For this review, take the finished solid that the model builds, in its own axes (mm). Give positions to 0.01 mm unless a question says otherwise; leave off trailing zeros. Order: outer loops, then holes, each group sorted by start corner. A loop starts at its lowest first (then second) coordinate and runs counter-clockwise, first axis right, second up.
Item 1: Consider section C-C (y = 136). Give the boundary of the cut face in (x, z).
Item 2: Consider section A-A (x = -201.93). Give the boundary of the cut face in (y, z).
Item 3: Consider section B-B (y = 90.5). Give the boundary of the cut face in (x, z), plus the area to 3 significant figures.
Item 4: Consider section D-D (x = -115). Give the boundary of the cut face in (y, z).
Item 5: For probe 1 along Y at (x, z) = (-151.13, 1.85); probe 2 along Y at (x, z) = (-74.93, 1.95); probe 3 along X at (y, z) = (216, 0.95), list the stretches that pass through material, from the lowest coordinate up.
```python
from build123d import *

# Parameters (mm, degrees)
SKETCH1_W               = 228.6
SKETCH1_H               = 228.6
BOSS_EXTRUDE1_DEPTH     = 2.54
SKETCH4_R               = 19.05
CUT_EXTRUDE2_DEPTH      = 378.179309613
FILL_PATTERN2_OUTLINE_R = 19.05
FILL_PATTERN2_DEPTH     = 2.54


# Read off the part's stored shape, not the designer's step: Fill Pattern2
with BuildPart() as part:
    # Sketch1 → Boss-Extrude1 (new body)
    with BuildSketch(Plane.XY):
        with Locations((-152.4, 152.4)):
            Rectangle(SKETCH1_W, SKETCH1_H)
    extrude(amount=BOSS_EXTRUDE1_DEPTH)

    # Sketch4 → Cut-Extrude2 (cut, through all)
    with BuildSketch(Plane.XY):
        with Locations((-227.33, 218.44)):
            Circle(SKETCH4_R)
    extrude(amount=CUT_EXTRUDE2_DEPTH, mode=Mode.SUBTRACT)

    # Fill Pattern2 outline → Fill Pattern2 (cut)
    with BuildSketch(Plane.XY):
        with Locations((-74.93, 130.451818976)):
            Circle(FILL_PATTERN2_OUTLINE_R)
        with Locations((-201.93, 86.457728463)):
            Circle(FILL_PATTERN2_OUTLINE_R)
        with Locations((-176.53, 218.44)):
            Circle(FILL_PATTERN2_OUTLINE_R)
        with Locations((-201.93, 174.445909488)):
            Circle(FILL_PATTERN2_OUTLINE_R)
        with Locations((-227.33, 130.451818976)):
            Circle(FILL_PATTERN2_OUTLINE_R)
        with Locations((-125.73, 130.451818976)):
            Circle(FILL_PATTERN2_OUTLINE_R)
        with Locations((-100.33, 174.445909488)):
            Circle(FILL_PATTERN2_OUTLINE_R)
        with Locations((-74.93, 218.44)):
            Circle(FILL_PATTERN2_OUTLINE_R)
        with Locations((-100.33, 86.457728463)):
            Circle(FILL_PATTERN2_OUTLINE_R)
        with Locations((-176.53, 130.451818976)):
            Circle(FILL_PATTERN2_OUTLINE_R)
        with Locations((-151.13, 174.445909488)):
            Circle(FILL_PATTERN2_OUTLINE_R)
        with Locations((-125.73, 218.44)):
            Circle(FILL_PATTERN2_OUTLINE_R)
        with Locations((-151.13, 86.457728463)):
            Circle(FILL_PATTERN2_OUTLINE_R)
    extrude(amount=FILL_PATTERN2_DEPTH, mode=Mode.SUBTRACT)


solid = part.part
```
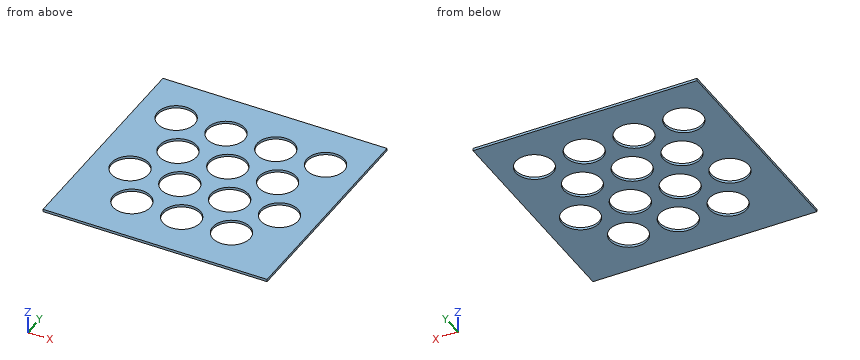
Resolved:
1. outline: (-266.7, 0) - (-245.55, 0) - (-245.55, 2.54) - (-266.7, 2.54) - close; (-209.11, 0) - (-194.75, 0) - (-194.75, 2.54) - (-209.11, 2.54) - close; (-158.31, 0) - (-143.95, 0) - (-143.95, 2.54) - (-158.31, 2.54) - close; (-107.51, 0) - (-93.15, 0) - (-93.15, 2.54) - (-107.51, 2.54) - close; (-56.71, 0) - (-38.1, 0) - (-38.1, 2.54) - (-56.71, 2.54) - close
2. outline: (38.1, 0) - (67.41, 0) - (67.41, 2.54) - (38.1, 2.54) - close; (105.51, 0) - (155.4, 0) - (155.4, 2.54) - (105.51, 2.54) - close; (193.5, 0) - (266.7, 0) - (266.7, 2.54) - (193.5, 2.54) - close
3. outline: (-266.7, 0) - (-220.55, 0) - (-220.55, 2.54) - (-266.7, 2.54) - close; (-183.31, 0) - (-169.75, 0) - (-169.75, 2.54) - (-183.31, 2.54) - close; (-132.51, 0) - (-118.95, 0) - (-118.95, 2.54) - (-132.51, 2.54) - close; (-81.71, 0) - (-38.1, 0) - (-38.1, 2.54) - (-81.71, 2.54) - close
3. area: 297 mm2
4. outline: (38.1, 0) - (74.3, 0) - (74.3, 2.54) - (38.1, 2.54) - close; (98.61, 0) - (114.71, 0) - (114.71, 2.54) - (98.61, 2.54) - close; (146.19, 0) - (162.29, 0) - (162.29, 2.54) - (146.19, 2.54) - close; (186.6, 0) - (202.7, 0) - (202.7, 2.54) - (186.6, 2.54) - close; (234.18, 0) - (266.7, 0) - (266.7, 2.54) - (234.18, 2.54) - close
5. probe 1: y = 38.1 to 67.41, 105.51 to 155.4, 193.5 to 266.7
5. probe 2: y = 38.1 to 111.4, 149.5 to 199.39, 237.49 to 266.7
5. probe 3: x = -266.7 to -246.22, -208.44 to -195.42, -157.64 to -144.62, -106.84 to -93.82, -56.04 to -38.1
